Could you check a few things on this model? Use its own coordinates, in mm. Face numbers are marked on the shaded views. A direction names the side the tool comes from. Give positions to 0.01 mm unless a question says otherwise; leave off trailing zeros. Loops run counter-clockwise (first coordinate to the right, second up) from the corner with the lowest first, then second, coordinate; pieces in that order, holes last. Notation, with made-up numbers: (-19.5, 25) -> (-10.5, 25) arc R19 ccw to (-10.5, 62) -> close; hole circle Ø4 at (12.5, -8.75). An arc over 180 degrees is marked (long way). Put each result on its own line as item: value.
Autodesk Fusion 360 part; units mm, degrees
sketch "Sketch1" plane through (0, 0, 0) normal (0, 0, 1) x (1, 0, 0)
  circle A0 centre (0, 0) radius 34.5
  line L0 (0, 0) -> (12, 0)
  line L1 (0, 0) -> (-6, 10.3923)
  line L2 (0, 0) -> (12, 0) construction
  line L3 (0, 0) -> (-6, -10.3923)
  line L4 (0, 0) -> (12, 0) construction
  circle A1 centre (-6, 10.3923) radius 9.5
  circle A2 centre (12, 0) radius 9.5
  circle A3 centre (-6, -10.3923) radius 9.5
  dimension "d1" = 69
  dimension "d2" = 12
  dimension "d3" = 12
  dimension "d4" = 120
  dimension "d5" = 120
  dimension "d6" = 12
  dimension "d7" = 19
  dimension "d8" = 19
  dimension "d9" = 19
extrude "Extrude1" add sketch "Sketch1" along normal blind 100
extrude "Extrude2" add sketch "Sketch1" along normal blind 20 contours A2 | A1 | A3
extrude "Extrude3" cut 1 faces at (10.3664, -17.9552, 100) along direction (0, 0, -1) blind 30
extrude "Extrude4" add 1 faces at (10.3664, -17.9552, 70) along direction (0, 0, 1) blind 20
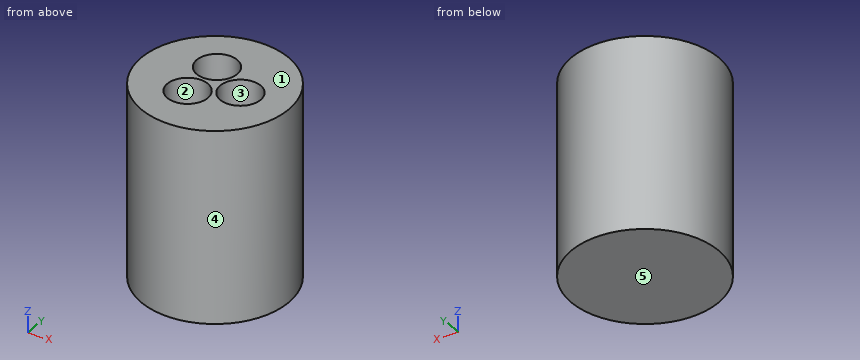
1. If we section it at A-A (y = 3.5): List the corners of the cut face in (x, z) for me.
Recorded:
outline: (-34.32, 0) -> (34.32, 0) -> (34.32, 90) -> (20.83, 90) -> (20.83, 20) -> (3.17, 20) -> (3.17, 90) -> (0.54, 90) -> (0.54, 20) -> (-12.54, 20) -> (-12.54, 90) -> (-34.32, 90) -> close
2. For the marked faces 1 and 2, which set-ups out of +Z, -Z, +X, -X, +Y, -Y let a thin tool reach every point of the face, with its end or its side?
Recorded:
face 1: +Z, +X, -X, +Y, -Y
face 2: +Z
3. If we section it at B-B (x = 12): List the corners of the cut face in (y, z) for me.
Recorded:
outline: (-32.35, 0) -> (32.35, 0) -> (32.35, 90) -> (9.5, 90) -> (9.5, 20) -> (-9.5, 20) -> (-9.5, 90) -> (-32.35, 90) -> close
4. Thinking about a two-plate mould opening in Y: for the marked faces 3, 4 and 5, which applies, pulls with the +Y half, pulls with the -Y half, needs draft (parallel to the pull), parting line crosses it, or undercut?
Recorded:
face 3: undercut
face 4: parting line crosses it
face 5: needs draft
5. If we section it at C-C (z = 16): List the corners of the cut face in (x, y) for me.
Recorded:
outline: circle Ø69 at (0, 0)
6. If we section it at D-D (z = 30): List the corners of the cut face in (x, y) for me.
Recorded:
outline: circle Ø69 at (0, 0); hole circle Ø19 at (-6, -10.39); hole circle Ø19 at (-6, 10.39); hole circle Ø19 at (12, 0)
7. I need wall thicknesses on line 1 (X direction, y = 6.5, z = 35.5); line 2 (Y direction, x = -14.5, z = 40.5); line 3 (Y direction, x = -8, z = 72). Which ranges of each line are inside material? Lowest first, please.
Recorded:
line 1: x = -33.88 to -14.67, 2.67 to 5.07, 18.93 to 33.88
line 2: y = -31.3 to -14.63, -6.15 to 6.15, 14.63 to 31.3
line 3: y = -33.56 to -19.68, -1.11 to 1.11, 19.68 to 33.56
8. I'm going to push flat-ended pins straight in: pin 1 (1 mm diameter, centred on y = -11.5, z = 32, fed in from -X); pin 2 (15 mm diameter, centred on x = -6, y = -10.39, fed in from +Z); pin 3 (8 mm diameter, centred on y = -20, z = 74.5, fed in from +X). Where does each tip first touch, or does it pass through?
Recorded:
pin 1: stops at x = -32.7
pin 2: stops at z = 20
pin 3: stops at x = 30.57
